Design review of the part built by this model. Coordinates are the model's own, in mm. A direction names the side the tool comes from. Coordinates: 2 decimals unless noted, no trailing zeros. Loops run counter-clockwise (first coordinate to the right, second up) from the corner with the lowest first, then second, coordinate; pieces in that order, holes last.
from build123d import *

# Parameters (mm, degrees)
EXTRUDE_1_DEPTH     = 4
CUT_EXTRUDE_1_DEPTH = 1.5
SKETCH_2_R          = 4
EXTRUDE_2_DEPTH     = 30
CUT_EXTRUDE_2_DEPTH = 5
CHAMFER_2_SIZE      = 1


with BuildPart() as part:
    # Эскиз1 → Бобышка-Вытянуть1 (new body, symmetric)
    with BuildSketch(Plane.XY):
        Polygon((8.9, 0), (-8.9, 0), (-8.9, 4), (-4, 4), (-4, 5.5), (4, 5.5), (4, 4), (8.9, 4), align=None)
    extrude(amount=EXTRUDE_1_DEPTH, both=True)

    # Эскиз3 → Вырез-Вытянуть1 (cut)
    with BuildSketch(Plane(origin=(0, 5.5, 0), x_dir=(1, 0, 0), z_dir=(0, 1, 0))):
        with BuildLine():
            Line((-4, 0), (-4, 4))
            Line((-4, 4), (0, 4))
            ThreePointArc((0, 4), (-2.828427125, 2.828427125), (-4, 0))
        make_face()
        with BuildLine():
            Line((0, -4), (4, -4))
            Line((4, -4), (4, 0))
            ThreePointArc((4, 0), (2.828427125, -2.828427125), (0, -4))
        make_face()
    extrude(amount=-CUT_EXTRUDE_1_DEPTH, mode=Mode.SUBTRACT)

    # Эскиз2 → Бобышка-Вытянуть2 (add)
    with BuildSketch(Plane(origin=(0, 5.5, 0), x_dir=(1, 0, 0), z_dir=(0, 1, 0))):
        with Locations(Location((0, 0, 0), (0, 0, 270))):  # turned: the seam where the file's is
            Circle(SKETCH_2_R)
    extrude(amount=EXTRUDE_2_DEPTH)

    # Эскиз4 → Вырез-Вытянуть2 (cut, through all)
    with BuildSketch(Plane(origin=(0, 4, 0), x_dir=(1, 0, 0), z_dir=(0, 1, 0))):
        with BuildLine():
            Line((-7.950471684, 4), (-8.9, 4))
            Line((-8.9, 4), (-8.9, 0))
            ThreePointArc((-8.9, 0), (-8.659364815, 2.055578022), (-7.950471684, 4))
        make_face()
        with BuildLine():
            Line((7.950471684, -4), (8.9, -4))
            Line((8.9, -4), (8.9, 0))
            ThreePointArc((8.9, 0), (8.659364815, -2.055578022), (7.950471684, -4))
        make_face()
    extrude(amount=-CUT_EXTRUDE_2_DEPTH, mode=Mode.SUBTRACT)

    # Вырез-По траектории1: sweep along a path in Эскиз6
    with BuildLine(Plane.XZ) as sweep_1_path:
        Line((0, -8.9), (8.9, -8.9))
        Line((8.9, -8.9), (8.9, 0))
        ThreePointArc((8.9, 0), (6.293250353, 6.293250353), (0, 8.9))
        Line((0, 8.9), (-8.9, 8.9))
        Line((-8.9, 8.9), (-8.9, 0))
        ThreePointArc((-8.9, 0), (-6.293250353, -6.293250353), (0, -8.9))
    # Эскиз5 → Вырез-По траектории1 (sweep, cut)
    with BuildSketch(Plane.XY.offset(4)):
        Polygon((-8.9, 2.5), (-4.8, 0), (-8.9, 0), align=None)
    sweep(path=sweep_1_path.line, transition=Transition.RIGHT, mode=Mode.SUBTRACT)

    # Фаска2
    chamfer_2_edges = [part.edges().sort_by_distance(p)[0] for p in [
        (0, 35.5, -4),
    ]]
    chamfer(chamfer_2_edges, length=CHAMFER_2_SIZE)


solid = part.part
Q1. Clearance check with flat-ended pins moving along their axes: pin 1 Ø0.8 at (y, z) = (5, -2.5) entering from +X; pin 2 Ø2.5 at (x, z) = (6.5, 0) entering from +Y; pin 3 Ø0.8 at (y, z) = (5, 2) entering from -X; pin 4 Ø1.5 at (x, y) = (5.5, 14) entering from -Z. State where each tip first meets the part, or that it passes through.
Q2. Machinability: for faces 1 (the flat face through (3, 5.5, -3)), 2 (the flat face through (4, 5, -2)), 3 (the flat face through (-4, 5, 2)), 4 (the flat face through (-3, 5.5, 3)), which of the approach directions +Z, -Z, +X, -X, +Y, -Y give a long, thin tool a straight path to every point of the face, cutting with its end or side? Answer none if there is none.
Q3. For line 1 (X direction, y = 22.5, z = -2.5); line 2 (Y direction, x = -4.5, z = -3); line 3 (Y direction, x = -7, z = -0.75), list the stretches that pass through material, from the lowest coordinate up.
Q4. Take a section at A-A, the plane y = 21. Write out the cut boundary in (x, z).
Entries:
1. pin 1: stops at x = 4
1. pin 2: stops at y = 4
1. pin 3: stops at x = -4
1. pin 4: passes through
2. face 1: -Z, +X, +Y
2. face 2: +Z, -Z, +X, +Y
2. face 3: +Z, -Z, -X, +Y
2. face 4: +Z, -X, +Y
3. line 1: x = -3.12 to 3.12
3. line 2: y = 0.37 to 4
3. line 3: y = 1.37 to 4
4. outline: circle Ø8 at (0, 0)
